Could you check a few things on this model? Use its own coordinates, in mm. Give positions to 0.01 mm unless a question says otherwise; leave off trailing zeros. Order: outer loops, then holes, each group sorted by start corner. A loop starts at its lowest first (then second) coordinate and runs counter-clockwise, first axis right, second up. Notation, with made-up numbers: (40, 72.25) -> (84, 72.25) arc R30 ccw to (84, 103.25) -> close; hole circle Ø3 at (83, 61.25). An arc over 180 degrees is marked (long way). Answer as CSV lines item,"result". Start each with the question number.
(1) I want a section at A-A (x = 0). Please give me the cut outline in (y, z) (1 decimal), plus the area to 3 significant figures.
(2) Will these pins go through, and if not, where does the flat tip stop? pin 1 Ø0.8 at (x, z) = (41.5, 0) entering from +Y; pin 2 Ø0.5 at (y, z) = (21.5, 0) entering from +X; pin 3 Ø9 at (x, y) = (0, -18.925) entering from +Z; pin 4 Ø0.8 at (y, z) = (-22.5, 0) entering from -X.
(3) I need wall thicknesses on L1, parallel to Y at x = 0, z = 0.05 (1 decimal); L2, parallel to Y at x = 55.5, z = 0.3; L3, parallel to Y at x = 3, z = -0.3 (1 decimal). Which ranges of each line are inside material? Lowest first, please.
(4) I want a section at C-C (x = 33). Please give me the cut outline in (y, z), plus the area to 3 significant figures.
```python
from build123d import *

# Parameters (mm, degrees)
SKETCH1_R           = 4
BOSS_EXTRUDE1_DEPTH = 0.79375


with BuildPart() as part:
    # Sketch1 → Boss-Extrude1 (new body, symmetric)
    with BuildSketch(Plane.XY):
        Polygon((25.4, -23.925), (25.4, -20.75), (71.12, -20.75), (71.12, 20.75), (25.4, 20.75), (25.4, 22.3375), (-25.4, 22.3375), (-25.4, 20.75), (-71.12, 20.75), (-71.12, -20.75), (-25.4, -20.75), (-25.4, -23.925), align=None)
        with Locations((0, -18.925)):
            Circle(SKETCH1_R, mode=Mode.SUBTRACT)
    extrude(amount=BOSS_EXTRUDE1_DEPTH, both=True)


solid = part.part
```
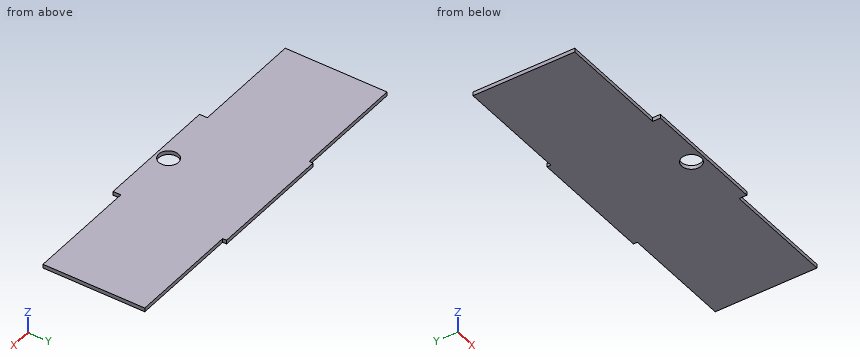
Final values:
1,outline,"(-23.9, -0.8) -> (-22.9, -0.8) -> (-22.9, 0.8) -> (-23.9, 0.8) -> close; (-14.9, -0.8) -> (22.3, -0.8) -> (22.3, 0.8) -> (-14.9, 0.8) -> close"
1,area,"60.7 mm²"
2,pin 1,"y = 20.75"
2,pin 2,"x = 25.4"
2,pin 3,"z = 0.79"
2,pin 4,"x = -25.4"
3,L1,"-23.9 to -22.9, -14.9 to 22.3"
3,L2,"-20.75 to 20.75"
3,L3,"-23.9 to -21.6, -16.3 to 22.3"
4,outline,"(-20.75, -0.79) -> (20.75, -0.79) -> (20.75, 0.79) -> (-20.75, 0.79) -> close"
4,area,"65.9 mm²"
